Work out the finished part from the listing and answer in its coordinate system (mm). A direction names the side the tool comes from. Coordinates: 2 decimals unless noted, no trailing zeros. Loops run counter-clockwise (first coordinate to the right, second up) from the corner with the lowest first, then second, coordinate; pieces in that order, holes last.
```python
from build123d import *

# Parameters (mm, degrees)
ESQUISSE1_W                    = 35
ESQUISSE1_H                    = 35
BOSS_EXTRU_1_DEPTH             = 14
CONG_1_R                       = 10
ESQUISSE2_R                    = 3
ENL_V_MAT_EXTRU_1_DEPTH        = 29.434134416
ENL_V_MAT_EXTRU_2_DEPTH        = 12
ESQUISSE4_W                    = 31.334316994
ESQUISSE4_H                    = 39.173265385
ENL_V_MAT_EXTRU_3_DEPTH        = 1.5
ENL_V_MAT_EXTRU_4_DEPTH        = 4
ESQUISSE6_W                    = 23.42
ESQUISSE6_H                    = 4
ENL_V_MAT_EXTRU_5_DEPTH        = 3.6
CONG_2_R                       = 3
ESQUISSE7_W                    = 19.75277675
ESQUISSE7_H                    = 6.328012926
ENL_V_MAT_EXTRU_6_DEPTH        = 6.5
ENL_V_MAT_EXTRU_7_DEPTH        = 28.504545079
ENL_V_MAT_EXTRU_7_DEPTH_BACK   = 28.504545079
ESQUISSE8_W                    = 25.702062378
ESQUISSE8_H                    = 0.5
ESQUISSE8_W_2                  = 29.01148979
ESQUISSE8_W_3                  = 33.519235733
BOSS_EXTRU_2_START             = 4
BOSS_EXTRU_2_DEPTH             = 4
BOSS_EXTRU_3_DEPTH             = 1.5
CHANFREIN1_SIZE                = 1.3
CONG_3_R                       = 3
BOSS_EXTRU_4_REACH             = 43.56
ESQUISSE11_W                   = 5.328012926
ESQUISSE11_H                   = 12.5
BOSS_EXTRU_4_DIRECTION_2_DEPTH = 2
CONG_4_R                       = 2
CONG_5_R                       = 2


with BuildPart() as part:
    # Esquisse1 → Boss.-Extru.1 (new body)
    with BuildSketch(Plane(origin=(0, 0, 0), x_dir=(1, 0, 0), z_dir=(0, 1, 0))):
        Rectangle(ESQUISSE1_W, ESQUISSE1_H)
    extrude(amount=BOSS_EXTRU_1_DEPTH)

    # Congé1
    cong_1_edges = [part.edges().sort_by_distance(p)[0] for p in [
        (17.5, 7, 17.5),
        (-17.5, 7, 17.5),
        (-17.5, 7, -17.5),
        (17.5, 7, -17.5),
    ]]
    fillet(cong_1_edges, radius=CONG_1_R)

    # Esquisse2 → Enlèv. mat.-Extru.1 (cut, through all)
    with BuildSketch(Plane(origin=(0, 14, 0), x_dir=(1, 0, 0), z_dir=(0, 1, 0))):
        with Locations(Location((0, 0, 0), (0, 0, 270))):
            Circle(ESQUISSE2_R)
    extrude(amount=-ENL_V_MAT_EXTRU_1_DEPTH, mode=Mode.SUBTRACT)

    # Esquisse3 → Enlèv. mat.-Extru.2 (cut)
    with BuildSketch(Plane(origin=(0, 14, 0), x_dir=(1, 0, 0), z_dir=(0, 1, 0))):
        Polygon((5.773502692, 0), (2.886751346, 5), (-2.886751346, 5), (-5.773502692, 0), (-2.886751346, -5), (2.886751346, -5), align=None)
    extrude(amount=-ENL_V_MAT_EXTRU_2_DEPTH, mode=Mode.SUBTRACT)

    # Esquisse4 → Enlèv. mat.-Extru.3 (cut)
    with BuildSketch(Plane(origin=(0, 14, 0), x_dir=(1, 0, 0), z_dir=(0, 1, 0))):
        with Locations((5.867158497, -0.053691428)):
            Rectangle(ESQUISSE4_W, ESQUISSE4_H)
    extrude(amount=-ENL_V_MAT_EXTRU_3_DEPTH, mode=Mode.SUBTRACT)

    # Esquisse5 → Enlèv. mat.-Extru.4 (cut)
    with BuildSketch(Plane(origin=(0, 12.5, 0), x_dir=(1, 0, 0), z_dir=(0, 1, 0))):
        with BuildLine():
            Line((-9.8, 11.71), (-9.8, -11.71))
            Line((-9.8, -11.71), (13.093327001, -14.049647704))
            ThreePointArc((13.093327001, -14.049647704), (16.180793539, -13.03910228), (17.5, -10.070374269))
            Line((17.5, -10.070374269), (17.5, 10.070374269))
            ThreePointArc((17.5, 10.070374269), (16.180793539, 13.03910228), (13.093327001, 14.049647704))
            Line((13.093327001, 14.049647704), (-9.8, 11.71))
        make_face()
    extrude(amount=-ENL_V_MAT_EXTRU_4_DEPTH, mode=Mode.SUBTRACT)

    # Esquisse6 → Enlèv. mat.-Extru.5 (cut)
    with BuildSketch(Plane(origin=(-9.8, 0, 0), x_dir=(0, 0, -1), z_dir=(1, 0, 0))):
        with Locations((0, 10.5)):
            Rectangle(ESQUISSE6_W, ESQUISSE6_H)
    extrude(amount=-ENL_V_MAT_EXTRU_5_DEPTH, mode=Mode.SUBTRACT)

    # Congé2
    cong_2_edges = [part.edges().sort_by_distance(p)[0] for p in [
        (-13.4, 12.5, 0),
    ]]
    fillet(cong_2_edges, radius=CONG_2_R)

    # Esquisse7 → Enlèv. mat.-Extru.6 (cut)
    with BuildSketch(Plane(origin=(0, 8.5, 0), x_dir=(1, 0, 0), z_dir=(0, 1, 0))):
        with Locations((6.123611625, -9.164006463)):
            Rectangle(ESQUISSE7_W, ESQUISSE7_H)
        with Locations((6.123611625, 9.164006463)):
            Rectangle(ESQUISSE7_W, ESQUISSE7_H)
    extrude(amount=-ENL_V_MAT_EXTRU_6_DEPTH, mode=Mode.SUBTRACT)

    # Esquisse8 → Enlèv. mat.-Extru.7 (cut, two sides: drawn at the far end of the back side and taken through both)
    with BuildSketch(Plane(origin=(0, 2, 0), x_dir=(1, 0, 0), z_dir=(0, 1, 0)).offset(-ENL_V_MAT_EXTRU_7_DEPTH_BACK)):
        with Locations((9.098254439, 6.25)):
            Rectangle(ESQUISSE8_W, ESQUISSE8_H)
        with Locations((9.098254439, 12.078012926)):
            Rectangle(ESQUISSE8_W, ESQUISSE8_H)
        with Locations((10.752968145, -6.25)):
            Rectangle(ESQUISSE8_W_2, ESQUISSE8_H)
        with Locations((13.006841117, -12.078012926)):
            Rectangle(ESQUISSE8_W_3, ESQUISSE8_H)
    extrude(amount=ENL_V_MAT_EXTRU_7_DEPTH + ENL_V_MAT_EXTRU_7_DEPTH_BACK, mode=Mode.SUBTRACT)

    # Esquisse9 → Boss.-Extru.2 (add)
    with BuildSketch(Plane(origin=(0, 8.5, 0), x_dir=(1, 0, 0), z_dir=(0, 1, 0)).offset(BOSS_EXTRU_2_START)):
        with BuildLine():
            Line((17.5, -7.5), (17.5, -6.5))
            Line((17.5, -6.5), (16, -6.5))
            Line((16, -6.5), (16, -11.828012926))
            Line((16, -11.828012926), (16.514893461, -11.828012926))
            ThreePointArc((16.514893461, -11.828012926), (17.250613689, -9.719354116), (17.5, -7.5))
        make_face()
        with BuildLine():
            Line((17.5, 6.5), (17.5, 7.5))
            ThreePointArc((17.5, 7.5), (17.250613689, 9.719354116), (16.514893461, 11.828012926))
            Line((16.514893461, 11.828012926), (16, 11.828012926))
            Line((16, 11.828012926), (16, 6.5))
            Line((16, 6.5), (17.5, 6.5))
        make_face()
    extrude(amount=-BOSS_EXTRU_2_DEPTH)

    # Esquisse10 → Boss.-Extru.3 (add)
    with BuildSketch(Plane(origin=(0, 12.5, 0), x_dir=(1, 0, 0), z_dir=(0, 1, 0))):
        with BuildLine():
            Line((13.16, 11.828012926), (20.5, 11.828012926))
            ThreePointArc((20.5, 11.828012926), (23.328427125, 10.65644005), (24.5, 7.828012926))
            Line((24.5, 7.828012926), (24.5, -7.828012926))
            ThreePointArc((24.5, -7.828012926), (23.328427125, -10.65644005), (20.5, -11.828012926))
            Line((20.5, -11.828012926), (13.16, -11.828012926))
            Line((13.16, -11.828012926), (13.16, 11.828012926))
        make_face()
    extrude(amount=BOSS_EXTRU_3_DEPTH)

    # Chanfrein1
    chanfrein1_edges = [part.edges().sort_by_distance(p)[0] for p in [
        (13.16, 14, 0),
    ]]
    chamfer(chanfrein1_edges, length=CHANFREIN1_SIZE)

    # Congé3
    cong_3_edges = [part.edges().sort_by_distance(p)[0] for p in [
        (16, 2, 9.164006463),
        (16, 2, -9.164006463),
    ]]
    fillet(cong_3_edges, radius=CONG_3_R)

    # Esquisse11 → Boss.-Extru.4 (add, up to next)
    with BuildSketch(Plane(origin=(17.5, 0, 0), x_dir=(0, 0, -1), z_dir=(1, 0, 0)), mode=Mode.PRIVATE) as boss_extru_4_sk1:
        with Locations((-9.164006463, 6.25)):
            Rectangle(ESQUISSE11_W, ESQUISSE11_H)
    boss_extru_4_tool1 = extrude(boss_extru_4_sk1.sketch, amount=-BOSS_EXTRU_4_REACH, mode=Mode.PRIVATE) - part.part
    # Esquisse11 → Boss.-Extru.4 (add, up to next)
    with BuildSketch(Plane(origin=(17.5, 0, 0), x_dir=(0, 0, -1), z_dir=(1, 0, 0)), mode=Mode.PRIVATE) as boss_extru_4_sk2:
        with Locations((9.164006463, 6.25)):
            Rectangle(ESQUISSE11_W, ESQUISSE11_H)
    boss_extru_4_tool2 = extrude(boss_extru_4_sk2.sketch, amount=-BOSS_EXTRU_4_REACH, mode=Mode.PRIVATE) - part.part
    add(boss_extru_4_tool1.solids().sort_by_distance((17.5, 6.25, 9.164006))[0])
    add(boss_extru_4_tool2.solids().sort_by_distance((17.5, 6.25, -9.164006))[0])

    # Esquisse11 → Boss.-Extru.4 direction 2 (add)
    with BuildSketch(Plane(origin=(17.5, 0, 0), x_dir=(0, 0, -1), z_dir=(1, 0, 0))):
        with Locations((-9.164006463, 6.25)):
            Rectangle(ESQUISSE11_W, ESQUISSE11_H)
        with Locations((9.164006463, 6.25)):
            Rectangle(ESQUISSE11_W, ESQUISSE11_H)
    extrude(amount=BOSS_EXTRU_4_DIRECTION_2_DEPTH)

    # Congé4
    cong_4_edges = [part.edges().sort_by_distance(p)[0] for p in [
        (19.5, 12.5, -9.164006463),
        (19.5, 12.5, 9.164006463),
        (19.5, 0, -9.164006463),
        (19.5, 0, 9.164006463),
    ]]
    fillet(cong_4_edges, radius=CONG_4_R)

    # Congé5
    cong_5_edges = [part.edges().sort_by_distance(p)[0] for p in [
        (-3.75277675, 2, 9.164006463),
        (-3.75277675, 2, -9.164006463),
    ]]
    fillet(cong_5_edges, radius=CONG_5_R)


solid = part.part
```
1. Each of these flat-tipped pins is pushed along its axis until it touches: P1, Ø7, axis at x = 12, y = 8, coming from the -Z side; P2, Ø6, axis at y = 10, z = 9.5, coming from the -X side; P3, Ø1, axis at x = -10, y = 12.5, coming from the -Z side; P4, Ø1.8, axis at x = -11, y = 10, coming from the -Z side. Where does it stop, or does it pass through?
2. A cutting plane is placed at C-C, the plane z = 10. Give the vertices of the cut face in (x, y), then the cut area to 3 significant figures.
3. A cutting plane is placed at A-A, the plane x = 8. Give the vertices of the cut face in (y, z), then the cut area to 3 significant figures.
4. For faces 4 (the cylindrical face through (15.14, 2.9, 9.13)), 5 (the flat face through (19.5, 6, 9)), 6 (the cylindrical face through (14.29, 10.53, 13.99)), determine the directions among +Z, -Z, +X, -X, +Y, -Y from which every point of the face is accessible in a straight line to the end or side of a thin tool.
5. Determine the mould class of faces 1 (the flat face through (-4.31, 5.296, -2.535)), 2 (the flat face through (7, 4, -6)), 3 (the cylindrical face through (23.359, 13.3, 10.625)) for opening direction X: released by +X, released by -X, zero draft, split by the parting line, or undercut.
6. Straight lines are drawn through the part: probe 1 along Z at (x, y) = (1, 2.5); probe 2 along X at (y, z) = (6.5, 7); probe 3 along X at (y, z) = (1, 0). For each, find the intervals that lie inside material, in ascending order.
7. A cutting plane is placed at B-B, the plane y = 1.5. Give the vertices of the cut face in (x, z), then the cut area to 3 significant figures.
8. A cutting plane is placed at D-D, the plane x = 0. Count the separate pieces of the cut face and the enclosed holes in it, then the cut area to 3 significant figures.
Answers below:
1. P1: stops at z = -17.45
1. P2: stops at x = -17.5
1. P3: stops at z = -17.3
1. P4: stops at z = -17.16
2. outline: (-17.18, 0) - (17.5, 0) arc R2 ccw to (19.5, 2) - (19.5, 10.5) arc R2 cw to (21.5, 12.5) - (23.86, 12.5) - (23.86, 14) - (14.46, 14) - (13.16, 12.7) - (13.16, 12.5) - (16, 12.5) - (16, 5) arc R3 cw to (13, 2) - (-1.75, 2) arc R2 cw to (-3.75, 4) - (-3.75, 8.5) - (-13.4, 8.5) - (-13.4, 9.5) arc R3 cw to (-10.4, 12.5) - (-9.8, 12.5) - (-9.8, 14) - (-17.18, 14) - close
2. area: 244 mm2
3. outline: (0, -17.49) - (12.5, -17.49) - (12.5, -13.53) - (8.5, -13.53) - (8.5, -12.33) - (0, -12.33) - close; (0, -11.83) - (2, -11.83) - (2, -6.5) - (0, -6.5) - close; (0, -6) - (8.5, -6) - (8.5, 6) - (0, 6) - close; (0, 6.5) - (2, 6.5) - (2, 11.83) - (0, 11.83) - close; (0, 12.33) - (8.5, 12.33) - (8.5, 13.53) - (12.5, 13.53) - (12.5, 17.49) - (0, 17.49) - close
3. area: 243 mm2
4. face 4: none
4. face 5: +Z, -Z, +X, -Y
4. face 6: +Y
5. face 1: undercut
5. face 2: zero draft
5. face 3: released by +X
6. probe 1: z = -17.5 to -12.33, -6 to -5, 5 to 6, 12.33 to 17.5
6. probe 2: x = -17.5 to -3.75, 16 to 19.5
6. probe 3: x = -17.5 to -3, 3 to 17.5
7. outline: (-17.5, -7.5) arc R10 ccw to (-7.5, -17.5) - (7.5, -17.5) arc R10 ccw to (16.26, -12.33) - (-3.75, -12.33) - (-3.75, -11.83) - (19.44, -11.83) - (19.44, -6.5) - (-3.75, -6.5) - (-3.75, -6) - (17.5, -6) - (17.5, 6) - (-3.75, 6) - (-3.75, 6.5) - (19.44, 6.5) - (19.44, 11.83) - (-3.75, 11.83) - (-3.75, 12.33) - (16.26, 12.33) arc R10 ccw to (7.5, 17.5) - (-7.5, 17.5) arc R10 ccw to (-17.5, 7.5) - close; hole circle Ø6 at (0, 0)
7. area: 1,090 mm2
8. separate pieces: 6
8. enclosed holes: 0
8. area: 173 mm2
